Autodesk Inventor part; units mm, degrees
ref_plane "YZ Plane" through (0, 0, 0) normal (1, 0, 0) x (0, 1, 0)
ref_plane "XZ Plane" through (0, 0, 0) normal (0, 1, 0) x (-1, 0, 0)
ref_plane "XY Plane" through (0, 0, 0) normal (0, 0, 1) x (1, 0, 0)
sketch "Sketch1" plane through (0, 0, 0) normal (0, 0, 1) x (1, 0, 0)
  circle A0 centre (0, 0) radius 56
  circle A1 centre (0, 0) radius 105
  dimension "d22" = 112
  dimension "d23" = 210
extrude "Plate1" add sketch "Sketch1" along normal blind 4
sketch "Sketch5" plane through (0, 0, 4) normal (0, 0, 1) x (1, 0, 0)
  circle A0 centre (60.1041, 60.1041) radius 9
  circle A1 centre (0, 0) radius 85 construction
  line L0 (60.1041, 60.1041) -> (0, 0) construction
  line L1 (0, 0) -> (0, 85) construction
  dimension "d24" = 18
  dimension "d25" = 170
  dimension "d31" = 45
extrude "Cut1" cut sketch "Sketch5" against normal blind 4
pattern_circular "Circular Pattern1" count 4 over 360 about axis through (0, 0, 0) along (0, 0, 1) of "Cut1"
equation "\"d22\" = Flange_Tube_diam"
equation "\"d23\" = Flange_D_outer"
equation "\"d24\" = Flange_d_hole_diam"
equation "\"d25\" = Flange_D1_hole_center"
equation "\"d26\" = Thickness"
equation "\"d2\" = Thickness"
equation "\"BendReliefWidth\" = Thickness"
equation "\"BendReliefDepth\" = 0.5 * Thickness"
equation "\"CornerReliefSize\" = 4 * Thickness"
equation "\"MinimumRemnant\" = 2 * Thickness"
equation "\"TransitionRadius\" = BendRadius"
equation "\"JacobiRadiusSize\" = BendRadius"
equation "\"GapSize\" = Thickness"
equation "\"Flange_D_outer\" = 210"
equation "\"Flange_D1_hole_center\" = 170"
equation "\"Flange_d_hole_diam\" = 18"
equation "\"Flange_Tube_diam\" = 112"
properties part number "drain flange" material "Stainless Steel"
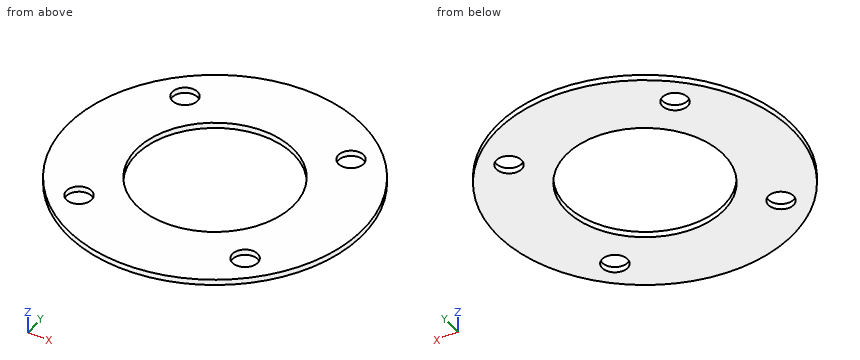
Build history of the part. All positions in model axes, mm. Give positions to 0.01 mm unless a question says otherwise; leave off trailing zeros. Loops run counter-clockwise (first coordinate to the right, second up) from the corner with the lowest first, then second, coordinate; pieces in that order, holes last. Notation, with made-up numbers: (-0.75, 19) -> (4.25, 19) arc R15 cw to (4.25, 29) -> close; hole circle Ø11 at (-33.5, 40). An arc over 180 degrees is marked (long way). Answer in a Markdown table with one row per item.
Item 1: Flat gauge pins, fed straight in: P1, Ø20.5, axis at x = -60.1, y = 60.1, coming from the -Z side; P2, Ø1, axis at x = -76.5, z = 3, coming from the -Y side. Where does each tip first touch, or does it go through?
Findings below:
| item | result |
|---|---|
| P1 | stops at z = 0 |
| P2 | stops at y = -72.45 |
Item 2: Slice it at C-C on z = 2.3. Write the cut outline in (x, y).
Findings below:
| item | result |
|---|---|
| outline | circle Ø210 at (0, 0); hole circle Ø18 at (-60.1, -60.1); hole circle Ø18 at (-60.1, 60.1); hole circle Ø112 at (0, 0); hole circle Ø18 at (60.1, -60.1); hole circle Ø18 at (60.1, 60.1) |
Item 3: Slice it at A-A on y = 0. Write the cut outline in (x, z), plus the area to 3 significant figures.
Findings below:
| item | result |
|---|---|
| outline | (-105, 0) -> (-56, 0) -> (-56, 4) -> (-105, 4) -> close; (56, 0) -> (105, 0) -> (105, 4) -> (56, 4) -> close |
| area | 392 mm² |
Item 4: Probe line 1 along Y through (x, z) = (64, 1.2); line 2 along Y through (x, z) = (-63, 0.3); line 3 along Y through (x, z) = (0, 2.9). List the from-to ranges inside material, lowest first. Write a range as [from, to].
Findings below:
| item | result |
|---|---|
| line 1 | y = [-83.24, -68.22], [-51.99, 51.99], [68.22, 83.24] |
| line 2 | y = [-84, -68.63], [-51.58, 51.58], [68.63, 84] |
| line 3 | y = [-105, -56], [56, 105] |
Item 5: Slice it at D-D on x = -76. Write the cut outline in (y, z).
Findings below:
| item | result |
|---|---|
| outline | (-72.45, 0) -> (72.45, 0) -> (72.45, 4) -> (-72.45, 4) -> close |
